```python
from build123d import *

# Parameters (mm, degrees)
BOSS_EXTRUDE1_DEPTH = 210.5
FILLET1_R           = 2


with BuildPart() as part:
    # Sketch1 → Boss-Extrude1 (new body)
    with BuildSketch(Plane.XY):
        with BuildLine():
            Line((0, 0), (-3.319764048, 5.75))
            ThreePointArc((-3.319764048, 5.75), (-3.319764048, 12.25), (2.309401077, 15.5))
            Line((2.309401077, 15.5), (96.309401077, 15.5))
            ThreePointArc((96.309401077, 15.5), (101.938566201, 12.25), (101.938566201, 5.75))
            Line((101.938566201, 5.75), (98.618802154, 0))
            Line((98.618802154, 0), (92.309401077, 0))
            Line((92.309401077, 0), (92.309401077, 2.75))
            ThreePointArc((92.309401077, 2.75), (86.309401077, 8.75), (80.309401077, 2.75))
            Line((80.309401077, 2.75), (80.309401077, 0))
            Line((80.309401077, 0), (38.359401077, 0))
            Line((38.359401077, 0), (38.359401077, 10))
            Line((38.359401077, 10), (26.259401077, 10))
            Line((26.259401077, 10), (26.259401077, 0))
            Line((26.259401077, 0), (18.309401077, 0))
            Line((18.309401077, 0), (18.309401077, 2.75))
            ThreePointArc((18.309401077, 2.75), (12.309401077, 8.75), (6.309401077, 2.75))
            Line((6.309401077, 2.75), (6.309401077, 0))
            Line((6.309401077, 0), (0, 0))
        make_face()
    extrude(amount=BOSS_EXTRUDE1_DEPTH)

    # Fillet1
    fillet1_edges = [part.edges().sort_by_distance(p)[0] for p in [
        (92.309401077, 0, 105.25),
        (80.309401077, 0, 105.25),
        (38.359401077, 0, 105.25),
        (26.259401077, 0, 105.25),
        (18.309401077, 0, 105.25),
        (6.309401077, 0, 105.25),
    ]]
    fillet(fillet1_edges, radius=FILLET1_R)


solid = part.part
```
Could you check a few things on this model? Use its own coordinates, in mm. A direction names the side the tool comes from. Round coordinates to 2 decimals unless told otherwise and drop trailing zeros. Loops run counter-clockwise (first coordinate to the right, second up) from the corner with the lowest first, then second, coordinate; pieces in that order, holes last. Notation, with made-up numbers: (64.25, 73) - (101.25, 73) arc R30 cw to (101.25, 96) - close; hole circle Ø4 at (-34.5, 84.5). An arc over 180 degrees is marked (long way). Answer in a Markdown table with one row per item. Add a question column.
(1) I'm going to push flat-ended pins straight in: pin 1 (1.5 mm diameter, centred on y = 10.5, z = 63.5, fed in from +X); pin 2 (0.6 mm diameter, centred on y = 2.5, z = 80.5, fed in from -X); pin 3 (3 mm diameter, centred on y = 1.5, z = 173.5, fed in from +X). Where does each tip first touch, or does it pass through?
(2) If we section it at A-A (z = 19): Please give me the cut outline in (x, y), plus the area to 3 significant figures.
(3) I need wall thicknesses on line 1 along X through (y, z) = (7.5, 32); line 2 along X through (y, z) = (6.75, 39); line 3 along Y through (x, z) = (97, 51). Which ranges of each line are inside material? Lowest first, please.
(4) If we mould it in two halves opening along X, with no side actions, what happens to faces 1 (the face through (50, 10, 210.5)), 2 (the face through (86.44, 8.75, 103.78)), 3 (the face through (-3.367, 12.167, 103.776))? For each: pulls with the +X half, pulls with the -X half, needs draft (parallel to the pull), parting line crosses it, or undercut.
(5) For faces 4 (the face through (50, 10, 0)), 5 (the face through (38.359, 6, 104)), which set-ups out of +Z, -Z, +X, -X, +Y, -Y let a thin tool reach every point of the face, with its end or its side?
(6) If we section it at B-B (x = 31.5): Please give me the cut outline in (y, z).
(7) If we section it at C-C (y = 12.5): Please give me the cut outline in (x, z), plus the area to 3 significant figures.
Model answer:
| question | item | result |
|---|---|---|
| 1 | pin 1 | stops at x = 102.77 |
| 1 | pin 2 | stops at x = -1.62 |
| 1 | pin 3 | stops at x = 100.35 |
| 2 | outline | (-3.32, 5.75) - (0, 0) - (4.31, 0) arc R2 ccw to (6.31, 2) - (6.31, 2.75) arc R6 cw to (18.31, 2.75) - (18.31, 2) arc R2 ccw to (20.31, 0) - (24.26, 0) arc R2 ccw to (26.26, 2) - (26.26, 10) - (38.36, 10) - (38.36, 2) arc R2 ccw to (40.36, 0) - (78.31, 0) arc R2 ccw to (80.31, 2) - (80.31, 2.75) arc R6 cw to (92.31, 2.75) - (92.31, 2) arc R2 ccw to (94.31, 0) - (98.62, 0) - (101.94, 5.75) arc R6.5 ccw to (96.31, 15.5) - (2.31, 15.5) arc R6.5 ccw to start |
| 2 | area | 1,300 mm² |
| 3 | line 1 | x = -4.02 to 8.64, 15.98 to 26.26, 38.36 to 82.64, 89.98 to 102.63 |
| 3 | line 2 | x = -3.79 to 7.84, 16.78 to 26.26, 38.36 to 81.84, 90.78 to 102.41 |
| 3 | line 3 | y = 0 to 15.46 |
| 4 | face 1 | needs draft |
| 4 | face 2 | undercut |
| 4 | face 3 | pulls with the -X half |
| 5 | face 4 | -Z, +X, -X, +Y, -Y |
| 5 | face 5 | +Z, -Z, -Y |
| 6 | outline | (10, 0) - (15.5, 0) - (15.5, 210.5) - (10, 210.5) - close |
| 7 | outline | (-3.17, 0) - (101.79, 0) - (101.79, 210.5) - (-3.17, 210.5) - close |
| 7 | area | 22,100 mm² |
